from build123d import *

# Parameters (mm, degrees)
F0_W      = 650
F0_H      = 1650
F0_W_2    = 500
F0_H_2    = 1400
F1_DEPTH  = 30
F5_D      = 5
F5_DEPTH  = 50
F5_TIP    = 1.5021515476
F7_D      = 5
F7_DEPTH  = 50
F7_TIP    = 1.5021515476
F10_D     = 5
F10_DEPTH = 15
F10_TIP   = 1.5021515476


with BuildPart() as f1:
    # F0 (on Front) → F1 (new body)
    with BuildSketch(Plane.XZ):
        Rectangle(F0_W, F0_H)
        Rectangle(F0_W_2, F0_H_2, mode=Mode.SUBTRACT)
    extrude(amount=F1_DEPTH)

    # F5
    with Locations(Plane(origin=(-325, 0, 0), x_dir=(0, -1, 0), z_dir=(-1, 0, 0))):
        with Locations((15, 795.0000119209), (15, 175.0000119209), (15, -794.9999880791)):
            Hole(F5_D / 2, depth=F5_DEPTH)
            with Locations((0, 0, -(F5_DEPTH + F5_TIP / 2))):  # 118° drill point
                Cone(0, F5_D / 2, F5_TIP, mode=Mode.SUBTRACT)

    # F7
    with Locations(Plane.YZ.offset(325)):
        with Locations((-14.9999763817, 795.000018446), (-14.9999763817, 175.000018446), (-14.9999763817, -794.999981554)):
            Hole(F7_D / 2, depth=F7_DEPTH)
            with Locations((0, 0, -(F7_DEPTH + F7_TIP / 2))):  # 118° drill point
                Cone(0, F7_D / 2, F7_TIP, mode=Mode.SUBTRACT)

    # F10
    with Locations(Plane.XY.offset(825)):
        with Locations((-295, -14.9999856949), (0, -15), (295, -15)):
            Hole(F10_D / 2, depth=F10_DEPTH)
            with Locations((0, 0, -(F10_DEPTH + F10_TIP / 2))):  # 118° drill point
                Cone(0, F10_D / 2, F10_TIP, mode=Mode.SUBTRACT)


solid = f1.part
Part model, mm, in its own coordinate system. A direction names the side the tool comes from. Coordinates: 2 decimals unless noted, no trailing zeros. Write each loop counter-clockwise with the first axis right and the second up, starting at its lowest first coordinate (ties: lowest second). Pieces come first, ordered by that corner, then holes. Notation, with made-up numbers: (-6, 2.5) - (28, 2.5) arc R33 cw to (28, 41.5) - close; hole circle Ø5 at (59, 54). An arc over 180 degrees is marked (long way). Put each result on its own line as item: value.
1. Band-saw the part on A-A (y = -23). Write the cut outline in (x, z).
Final values:
outline: (-325, -825) - (325, -825) - (325, 825) - (-325, 825) - close; hole (-250, -700) - (250, -700) - (250, 700) - (-250, 700) - close
2. Band-saw the part on C-C (x = -203.5). Write the cut outline in (y, z), then the cut area to 3 significant figures.
Final values:
outline: (-30, -825) - (0, -825) - (0, -700) - (-30, -700) - close; (-30, 700) - (0, 700) - (0, 825) - (-30, 825) - close
area: 7,500 mm²
3. Flat gauge pins, fed straight in: pin 1 Ø6.5 at (y, z) = (-15, -795) entering from -X; pin 2 Ø4 at (y, z) = (-15, 175) entering from +X; pin 3 Ø3 at (y, z) = (-15, 175) entering from -X; pin 4 Ø4 at (x, y) = (-295, -15) entering from +Z. Where does each tip first touch, or does it go through?
Final values:
pin 1: stops at x = -325
pin 2: stops at x = 274.7
pin 3: stops at x = -274.4
pin 4: stops at z = 809.7
4. Two-plate mould, pull along X, no slides. Class faces 1 (the flat face through (-3, -15, 700)), 2 (the flat face through (250, -15, -10)), 3 (the flat face through (284, 0, 12)), 4 (the flat face through (-325, -15, -12)): +X half, -X half, draft (parallel to the pull), parting line (faces both ways), or undercut.
Final values:
face 1: undercut
face 2: undercut
face 3: draft
face 4: -X half
5. Probe line 1 along Z through (x, y) = (-298.5, -15); line 2 along X through (y, z) = (-15.25, -667); line 3 along Z through (x, y) = (-164.5, -17.5). List the from-to ranges inside material, lowest first. Write a range as [from, to].
Final values:
line 1: z = [-825, -797.5], [-792.5, 172.5], [177.5, 792.5], [797.5, 825]
line 2: x = [-325, -250], [250, 325]
line 3: z = [-825, -700], [700, 825]
6. 3-axis set-ups, long thin cutter, end or side, ignore diameter. For faces 5 (the flat face through (284, -30, 12)), 6 (the flat face through (-3, -15, -700)): which of +Z, -Z, +X, -X, +Y, -Y reach the whole face in a straight line?
Final values:
face 5: +Z, -Z, +X, -X, -Y
face 6: +Y, -Y
7. Band-saw the part on B-B (z = -591.5). Write the cut outline in (x, y), then the cut area to 3 significant figures.
Final values:
outline: (-325, -30) - (-250, -30) - (-250, 0) - (-325, 0) - close; (250, -30) - (325, -30) - (325, 0) - (250, 0) - close
area: 4,500 mm²
